from build123d import *

# Parameters (mm, degrees)
SKIZZE1_W                       = 42.3
SKIZZE1_H                       = 42.3
AUFSATZ_LINEAR_AUSTRAGEN1_DEPTH = 40
SKIZZE2_R                       = 11
AUFSATZ_LINEAR_AUSTRAGEN2_DEPTH = 2
SKIZZE3_R                       = 2.5
AUFSATZ_LINEAR_AUSTRAGEN3_DEPTH = 22
SKIZZE4_W                       = 5
SKIZZE4_H                       = 0.5
SCHNITT_LINEAR_AUSTRAGEN1_DEPTH = 20
M3_GEWINDEBOHRUNG2_D            = 2.5
M3_GEWINDEBOHRUNG2_DEPTH        = 8.5
M3_GEWINDEBOHRUNG2_TIP          = 0.751075774
FASE6_SIZE                      = 5


with BuildPart() as part:
    # Skizze1 → Aufsatz-Linear austragen1 (new body)
    with BuildSketch(Plane.XY):
        with Locations((0.382196485, -6.777376721)):
            Rectangle(SKIZZE1_W, SKIZZE1_H)
    extrude(amount=AUFSATZ_LINEAR_AUSTRAGEN1_DEPTH)

    # Skizze2 → Aufsatz-Linear austragen2 (add)
    with BuildSketch(Plane.XY.offset(40)):
        with Locations((0.382196485, -6.777376721)):
            Circle(SKIZZE2_R)
    extrude(amount=AUFSATZ_LINEAR_AUSTRAGEN2_DEPTH)

    # Skizze3 → Aufsatz-Linear austragen3 (add)
    with BuildSketch(Plane.XY.offset(42)):
        with Locations((0.382196485, -6.777376721)):
            Circle(SKIZZE3_R)
    extrude(amount=AUFSATZ_LINEAR_AUSTRAGEN3_DEPTH)

    # Skizze4 → Schnitt-Linear austragen1 (cut)
    with BuildSketch(Plane.XY.offset(64)):
        with Locations((0.382196485, -4.527376721)):
            Rectangle(SKIZZE4_W, SKIZZE4_H)
    extrude(amount=-SCHNITT_LINEAR_AUSTRAGEN1_DEPTH, mode=Mode.SUBTRACT)

    # M3 Gewindebohrung2
    with Locations(Plane.XY.offset(40)):
        with Locations((-15.117803515, 8.722623279), (15.882196485, 8.722623279), (-15.117803515, -22.277376721), (15.882196485, -22.277376721)):
            Hole(M3_GEWINDEBOHRUNG2_D / 2, depth=M3_GEWINDEBOHRUNG2_DEPTH)
            with Locations((0, 0, -(M3_GEWINDEBOHRUNG2_DEPTH + M3_GEWINDEBOHRUNG2_TIP / 2))):  # 118° drill point
                Cone(0, M3_GEWINDEBOHRUNG2_D / 2, M3_GEWINDEBOHRUNG2_TIP, mode=Mode.SUBTRACT)

    # Fase6
    fase6_edges = [part.edges().sort_by_distance(p)[0] for p in [
        (-20.767803515, 14.372623279, 20),
        (21.532196485, 14.372623279, 20),
        (21.532196485, -27.927376721, 20),
        (-20.767803515, -27.927376721, 20),
    ]]
    chamfer(fase6_edges, length=FASE6_SIZE)


solid = part.part
Could you check a few things on this model? Use its own coordinates, in mm. A direction names the side the tool comes from. Round coordinates to 2 decimals unless told otherwise and drop trailing zeros. Loops run counter-clockwise (first coordinate to the right, second up) from the corner with the lowest first, then second, coordinate; pieces in that order, holes last. Notation, with made-up numbers: (50, 17.5) - (94, 17.5) arc R13 ccw to (94, 31.5) - close; hole circle Ø2 at (-39.75, 17.25). An arc over 180 degrees is marked (long way). Write item = value, one per line.
1) If we mould it in two halves opening along Y, with no side actions, what happens to faces 1 (the flat face through (-20.768, -7, 20)), 2 (the conical face through (-15.15, -22.06, 30.88)), 3 (the cylindrical face through (6.296, 2.498, 40.986)), 4 (the flat face through (19.07, -25.39, 19.72))? For each: pulls with the +Y half, pulls with the -Y half, needs draft (parallel to the pull), parting line crosses it, or undercut.
Computed:
face_1 = needs draft
face_2 = undercut
face_3 = parting line crosses it
face_4 = pulls with the -Y half
2) I need wall thicknesses on line 1 along X through (y, z) = (-23, 36.5); line 2 along Z through (x, y) = (14.5, -21); line 3 along Y through (x, z) = (17, 34). Which ranges of each line are inside material? Lowest first, please. Write a range as from..to.
Computed:
line_1 = -20.7..-16.14, -14.1..14.86, 16.9..21.46
line_2 = 0..40
line_3 = -27.46..-22.84, -21.72..8.16, 9.28..13.9
3) Imagine slicing it at C-C (y = -3). Please give me the cut outline in (x, z), and give its area (3 significant figures).
Computed:
outline = (-20.77, 0) - (21.53, 0) - (21.53, 40) - (10.71, 40) - (10.71, 42) - (-9.95, 42) - (-9.95, 40) - (-20.77, 40) - close
area = 1,730 mm2
4) On a 3-axis mill with a long thin cutter (end or side, diameter ignored), from which of +Z, -Z, +X, -X, +Y, -Y can I reach the whole of each face in a straight line? I mean faces 5 (the cylindrical face through (14.69, 9.1, 35.69)), 6 (the flat face through (21.532, -7, 20)), 7 (the flat face through (0, -4.777, 54)). Say none if no direction works.
Computed:
face_5 = +Z
face_6 = +Z, -Z, +X, +Y, -Y
face_7 = +Z, +X, -X, +Y
5) Imagine slicing it at D-D (x = 0). Please give me the cut outline in (y, z).
Computed:
outline = (-27.93, 0) - (14.37, 0) - (14.37, 40) - (4.22, 40) - (4.22, 42) - (-4.31, 42) - (-4.31, 44) - (-4.78, 44) - (-4.78, 64) - (-9.25, 64) - (-9.25, 42) - (-17.77, 42) - (-17.77, 40) - (-27.93, 40) - close
6) Imagine slicing it at B-B (z = 38). Please give me the cut outline in (x, y), and give its area (3 significant figures).
Computed:
outline = (-20.77, -22.93) - (-15.77, -27.93) - (16.53, -27.93) - (21.53, -22.93) - (21.53, 9.37) - (16.53, 14.37) - (-15.77, 14.37) - (-20.77, 9.37) - close; hole circle Ø2.5 at (-15.12, -22.28); hole circle Ø2.5 at (-15.12, 8.72); hole circle Ø2.5 at (15.88, -22.28); hole circle Ø2.5 at (15.88, 8.72)
area = 1,720 mm2
7) Imagine slicing it at A-A (z = 26). Please give me the cut outline in (x, y).
Computed:
outline = (-20.77, -22.93) - (-15.77, -27.93) - (16.53, -27.93) - (21.53, -22.93) - (21.53, 9.37) - (16.53, 14.37) - (-15.77, 14.37) - (-20.77, 9.37) - close
8) I'm going to push flat-ended pins straight in: P1, Ø1.5, axis at x = 15.88, y = -22.28, coming from the +Z side; P2, Ø4, axis at x = -2, y = -2.5, coming from the +Z side; P3, Ø2.5, axis at x = -0.5, z = 50, coming from the +Y side. Where does each tip first touch, or does it pass through?
Computed:
P1 = 31.2
P2 = 42
P3 = -4.78
